```python
from build123d import *

# Parameters (mm, degrees)
SKETCH2_W      = 50.8
SKETCH2_H      = 73.025
SKETCH2_R      = 3.175
EXTRUDE1_DEPTH = 9.525


with BuildPart() as part:
    # Sketch2 → Extrude1 (new body)
    with BuildSketch(Plane.XY):
        with Locations((25.4, 36.5125)):
            Rectangle(SKETCH2_W, SKETCH2_H)
        with Locations((12.7, 60.325)):
            Circle(SKETCH2_R, mode=Mode.SUBTRACT)
        with Locations((38.1, 60.325)):
            Circle(SKETCH2_R, mode=Mode.SUBTRACT)
        Polygon((31.815804866, 18.25625), (28.607902433, 23.8125), (22.192097567, 23.8125), (18.984195134, 18.25625), (22.192097567, 12.7), (28.607902433, 12.7), align=None, mode=Mode.SUBTRACT)
    extrude(amount=EXTRUDE1_DEPTH)


solid = part.part
```
The model under review builds one solid part; all positions refer to its coordinate system, in mm. A direction names the side the tool comes from. Give positions to 0.01 mm unless a question says otherwise; leave off trailing zeros. Write each loop counter-clockwise with the first axis right and the second up, starting at its lowest first coordinate (ties: lowest second). Pieces come first, ordered by that corner, then holes.
(1) Consider section C-C, the plane x = 11. Give the boundary of the cut face in (y, z) (3 decimals), and give its area (3 significant figures).
(2) The part is to be moulded in two halves that separate along Y. For faces 3 (the flat face through (25, 37, 9.525)), 4 (the cylindrical face through (12.287, 63.473, 4.696)), 5 (the flat face through (25, 0, 5)), say which applies: released by +Y, released by -Y, zero draft, split by the parting line, or undercut.
(3) To check wall thickness, follow L1, parallel to Y at x = 28, z = 2.5 (1 decimal); L2, parallel to Y at x = 38.1, z = 2.5 (3 decimals); L3, parallel to X at y = 18.5, z = 1.5. State the ranges of each line that lie inside material, in increasing order.
(4) Consider section B-B, the plane z = 4.5. Give the number of separate pieces and of enclosed holes in the cut face, and give its area (3 significant figures).
(5) Consider section A-A, the plane x = 38.1. Give the boundary of the cut face in (y, z) (3 decimals), and give its area (3 significant figures).
(6) Tool access review of faces 1 (the flat face through (25, 12.7, 5)), 2 (the flat face through (25, 73.025, 5)): name each direction out of +Z, -Z, +X, -X, +Y, -Y from which nothing blocks a thin tool from reaching the whole face with its end or side.
Returned:
1. outline: (0, 0) - (57.643, 0) - (57.643, 9.525) - (0, 9.525) - close; (63.007, 0) - (73.025, 0) - (73.025, 9.525) - (63.007, 9.525) - close
1. area: 644 mm2
2. face 3: zero draft
2. face 4: undercut
2. face 5: released by -Y
3. L1: y = 0 to 12.7, 23.8 to 73
3. L2: y = 0 to 57.15, 63.5 to 73.025
3. L3: x = 0 to 19.12, 31.68 to 50.8
4. separate pieces: 1
4. enclosed holes: 3
4. area: 3,540 mm2
5. outline: (0, 0) - (57.15, 0) - (57.15, 9.525) - (0, 9.525) - close; (63.5, 0) - (73.025, 0) - (73.025, 9.525) - (63.5, 9.525) - close
5. area: 635 mm2
6. face 1: +Z, -Z
6. face 2: +Z, -Z, +X, -X, +Y
